from build123d import *

# Parameters (mm, degrees)
SKETCH_1_R          = 10
EXTRUDE_1_DEPTH     = 21
SKETCH_2_R          = 40
EXTRUDE_2_DEPTH     = 5
CHAMFER_1_SIZE      = 10
SKETCH_3_R          = 2.75
CUT_EXTRUDE_2_DEPTH = 5
CHAMFER_2_SIZE      = 0.5
SKETCH_4_R          = 1.5
CUT_EXTRUDE_3_DEPTH = 63.257529665


with BuildPart() as part:
    # 草图1 → 凸台-拉伸1 (new body)
    with BuildSketch(Plane(origin=(0, 0, 0), x_dir=(1, 0, 0), z_dir=(0, 1, 0))):
        with Locations(Location((0, 0, 0), (0, 0, 90))):
            Circle(SKETCH_1_R)
        with BuildLine():
            Line((-1.734935157, 1.8), (1.734935157, 1.8))
            ThreePointArc((1.734935157, 1.8), (0, -2.5), (-1.734935157, 1.8))
        make_face(mode=Mode.SUBTRACT)
    extrude(amount=EXTRUDE_1_DEPTH)

    # 草图2 → 凸台-拉伸2 (add)
    with BuildSketch(Plane(origin=(0, 21, 0), x_dir=(1, 0, 0), z_dir=(0, 1, 0))):
        with Locations(Location((0, 0, 0), (0, 0, 270))):
            Circle(SKETCH_2_R)
    extrude(amount=EXTRUDE_2_DEPTH)

    # 倒角1
    chamfer_1_edges = [part.edges().sort_by_distance(p)[0] for p in [
        (0, 21, 10),
    ]]
    chamfer(chamfer_1_edges, length=CHAMFER_1_SIZE)

    # 草图3 → 切除-拉伸2 (cut)
    with BuildSketch(Plane(origin=(0, 26, 0), x_dir=(1, 0, 0), z_dir=(0, 1, 0))):
        with Locations(Location((0, 30, 0), (0, 0, 270))):
            Circle(SKETCH_3_R)
        with Locations(Location((30, 0, 0), (0, 0, 270))):
            Circle(SKETCH_3_R)
        with Locations(Location((0, -30, 0), (0, 0, 270))):
            Circle(SKETCH_3_R)
        with Locations(Location((-30, 0, 0), (0, 0, 270))):
            Circle(SKETCH_3_R)
    extrude(amount=-CUT_EXTRUDE_2_DEPTH, mode=Mode.SUBTRACT)

    # 倒角2
    chamfer_2_edges = [part.edges().sort_by_distance(p)[0] for p in [
        (0, 26, -32.75),
        (30, 26, -2.75),
        (0, 26, 27.25),
        (-30, 26, -2.75),
    ]]
    chamfer(chamfer_2_edges, length=CHAMFER_2_SIZE)

    # 草图4 → 切除-拉伸3 (cut, through all)
    with BuildSketch(Plane.XY):
        with Locations((0, 16.5)):
            Circle(SKETCH_4_R)
    extrude(amount=-CUT_EXTRUDE_3_DEPTH, mode=Mode.SUBTRACT)


solid = part.part
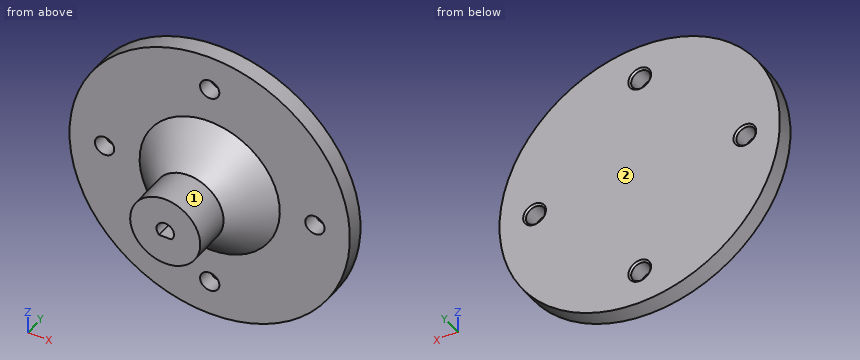
CAD build for the part. Positions are in the model's coordinates, mm. Face numbers are marked on the shaded views. A direction names the side the tool comes from. Round coordinates to 2 decimals unless told otherwise and drop trailing zeros. Loops run counter-clockwise (first coordinate to the right, second up) from the corner with the lowest first, then second, coordinate; pieces in that order, holes last. Notation, with made-up numbers: M 68.5,-0.5 L 90.5,-0.5 A10 ccw 90.5,4.5 Z; hole C 56.25,77.5 d2. An arc over 180 degrees is marked long. One line per question, with ' | ' between items. Start each with the question number.
Item 1: Which spindle directions (+Z, -Z, +X, -X, +Y, -Y) get a long thin tool onto all of the face, cutting with end or side? Do the marked faces 1 and 2. Say none if no direction does.
Item 2: Cut at D-D, the plane y = 19.25. Write the cut outline in (x, z), plus the area to 3 significant figures.
Item 3: Cut at A-A, the plane z = 0. Write the cut outline in (x, y).
Item 4: Pin check, flat tips, straight feed: pin 1 Ø2 at (x, z) = (-0.5, 1) entering from -Y; pin 2 Ø5 at (x, z) = (-30, 0) entering from -Y; pin 3 Ø1.5 at (y, z) = (17.5, -12) entering from -X; pin 4 Ø1.8 at (x, y) = (0, 16.5) entering from +Z. Stop position of each tip, or through.
Item 5: Wall check: line 1 (X direction, y = 24.3, z = 0); line 2 (X direction, y = 5.5, z = 0); line 3 (Y direction, x = -1.5, z = -20). Give the ranges that are in metal, low to high.
Item 6: Cut at B-B, the plane x = 0. State how many separate pieces and enclosed holes the cut face has, plus the area to 3 significant figures.
Item 7: Cut at C-C, the plane x = -30. Write the cut outline in (y, z).
Responses:
1) face 1: -Y | face 2: +Z, -Z, +X, -X, +Y
2) outline: C 0,0 d36.5; hole M -1.73,-1.8 L 1.73,-1.8 A2.5 ccw long Z | area: 1,030 mm²
3) outline: M -40,21 L -32.75,21 L -32.75,25.5 L -33.25,26 L -40,26 Z; M -27.25,21 L -20,21 L -10,11 L -10,0 L -2.5,0 L -2.5,21 L 2.5,21 L 2.5,0 L 10,0 L 10,11 L 20,21 L 27.25,21 L 27.25,25.5 L 26.75,26 L -26.75,26 L -27.25,25.5 Z; M 32.75,21 L 40,21 L 40,26 L 33.25,26 L 32.75,25.5 Z
4) pin 1: stops at y = 21 | pin 2: passes through | pin 3: stops at x = -12.61 | pin 4: stops at z = 16.4
5) line 1: x = -40 to -32.75, -27.25 to 27.25, 32.75 to 40 | line 2: x = -10 to -2.5, 2.5 to 10 | line 3: y = 21 to 26
6) separate pieces: 4 | enclosed holes: 0 | area: 733 mm²
7) outline: M 21,-26.46 L 26,-26.46 L 26,-3.25 L 25.5,-2.75 L 21,-2.75 Z; M 21,2.75 L 25.5,2.75 L 26,3.25 L 26,26.46 L 21,26.46 Z
